For this review, take the finished solid that the model builds, in its own axes (mm). A direction names the side the tool comes from. Coordinates: 2 decimals unless noted, no trailing zeros. Write each loop counter-clockwise with the first axis right and the second up, starting at its lowest first coordinate (ties: lowest second). Pieces come first, ordered by that corner, then holes.
```python
from build123d import *

# Parameters (mm, degrees)
SKETCH_R      = 3
SKETCH_R_2    = 2.1
SKETCH_R_3    = 20
PAD_DEPTH     = 12
SKETCH001_R   = 40
SKETCH001_R_2 = 30
POCKET_DEPTH  = 8


with BuildPart() as part:
    # Sketch → Pad (new body)
    with BuildSketch(Plane.XY):
        with BuildLine():
            ThreePointArc((-37.373806, -14.254775), (0, -40), (37.373806, -14.254775))
            ThreePointArc((39.685017, -5.009931), (35.149287, -8.787322), (37.373806, -14.254775))
            ThreePointArc((39.685017, -5.009931), (0, 40), (-39.685017, -5.009931))
            ThreePointArc((-37.373806, -14.254775), (-35.149287, -8.787322), (-39.685017, -5.009931))
        make_face()
        with Locations((0, 35)):
            Circle(SKETCH_R, mode=Mode.SUBTRACT)
        with Locations((-30.310889, -17.5)):
            Circle(SKETCH_R, mode=Mode.SUBTRACT)
        with Locations((30.310889, -17.5)):
            Circle(SKETCH_R, mode=Mode.SUBTRACT)
        with Locations((-22.51666, 13)):
            Circle(SKETCH_R_2, mode=Mode.SUBTRACT)
        with Locations((22.51666, 13)):
            Circle(SKETCH_R_2, mode=Mode.SUBTRACT)
        with Locations((0, -26)):
            Circle(SKETCH_R_2, mode=Mode.SUBTRACT)
        Circle(SKETCH_R_3, mode=Mode.SUBTRACT)
    extrude(amount=PAD_DEPTH)

    # Sketch001 (on Face13 of Pad) → Pocket (cut)
    with BuildSketch(Plane.XY.offset(12)):
        Circle(SKETCH001_R)
        Circle(SKETCH001_R_2, mode=Mode.SUBTRACT)
    extrude(amount=-POCKET_DEPTH, mode=Mode.SUBTRACT)


solid = part.part
```
Q1. Add section A-A (y = 0). State the section outline as (x, z) points.
Ans:
outline: (-40, 0) - (-20, 0) - (-20, 12) - (-30, 12) - (-30, 4) - (-40, 4) - close; (20, 0) - (40, 0) - (40, 4) - (30, 4) - (30, 12) - (20, 12) - close
Q2. Add section B-B (x = 0). State the section outline as (y, z) points.
Ans:
outline: (-40, 0) - (-28.1, 0) - (-28.1, 12) - (-30, 12) - (-30, 4) - (-40, 4) - close; (-23.9, 0) - (-20, 0) - (-20, 12) - (-23.9, 12) - close; (20, 0) - (32, 0) - (32, 4) - (30, 4) - (30, 12) - (20, 12) - close; (38, 0) - (40, 0) - (40, 4) - (38, 4) - close
Q3. For probe 1 along Y at (x, z) = (0, 5); probe 2 along Y at (x, z) = (-1, 5.5); probe 3 along X at (y, z) = (7, 9) (3 decimals), list the stretches that pass through material, from the lowest coordinate up.
Ans:
probe 1: y = -30 to -28.1, -23.9 to -20, 20 to 30
probe 2: y = -29.98 to -27.85, -24.15 to -19.97, 19.97 to 29.98
probe 3: x = -29.172 to -18.735, 18.735 to 29.172
Q4. Tool access review of faces 1 (the cylindrical face through (-29.97, 1.32, 8.06)), 2 (the cylindrical face through (-20.514, 13.631, 5.916)): name each direction out of +Z, -Z, +X, -X, +Y, -Y from which nothing blocks a thin tool from reaching the whole face with its end or side.
Ans:
face 1: +Z
face 2: +Z, -Z
Q5. Add section D-D (z = 10). State the section outline as (x, y) points, then the cut area to 3 significant figures.
Ans:
outline: circle Ø60 at (0, 0); hole circle Ø4.2 at (-22.52, 13); hole circle Ø40 at (0, 0); hole circle Ø4.2 at (0, -26); hole circle Ø4.2 at (22.52, 13)
area: 1,530 mm2
Q6. Add section C-C (z = 2.25). State the section outline as (x, y) points.
Ans:
outline: (-39.69, -5.01) arc R5 cw to (-37.37, -14.25) arc R40 ccw to (37.37, -14.25) arc R5 cw to (39.69, -5.01) arc R40 ccw (long way) to start; hole circle Ø6 at (-30.31, -17.5); hole circle Ø4.2 at (-22.52, 13); hole circle Ø40 at (0, 0); hole circle Ø6 at (0, 35); hole circle Ø4.2 at (0, -26); hole circle Ø4.2 at (22.52, 13); hole circle Ø6 at (30.31, -17.5)
Q7. Clearance check with flat-ended pins moving along their axes: pin 1 Ø5 at (y, z) = (20.5, 2) entering from +X; pin 2 Ø1.5 at (y, z) = (-23.5, 9) entering from -X; pin 3 Ø4 at (x, z) = (8, 2) entering from +Y. State where each tip first meets the part, or that it passes through.
Ans:
pin 1: stops at x = 35.72
pin 2: stops at x = -19.56
pin 3: stops at y = 39.55
